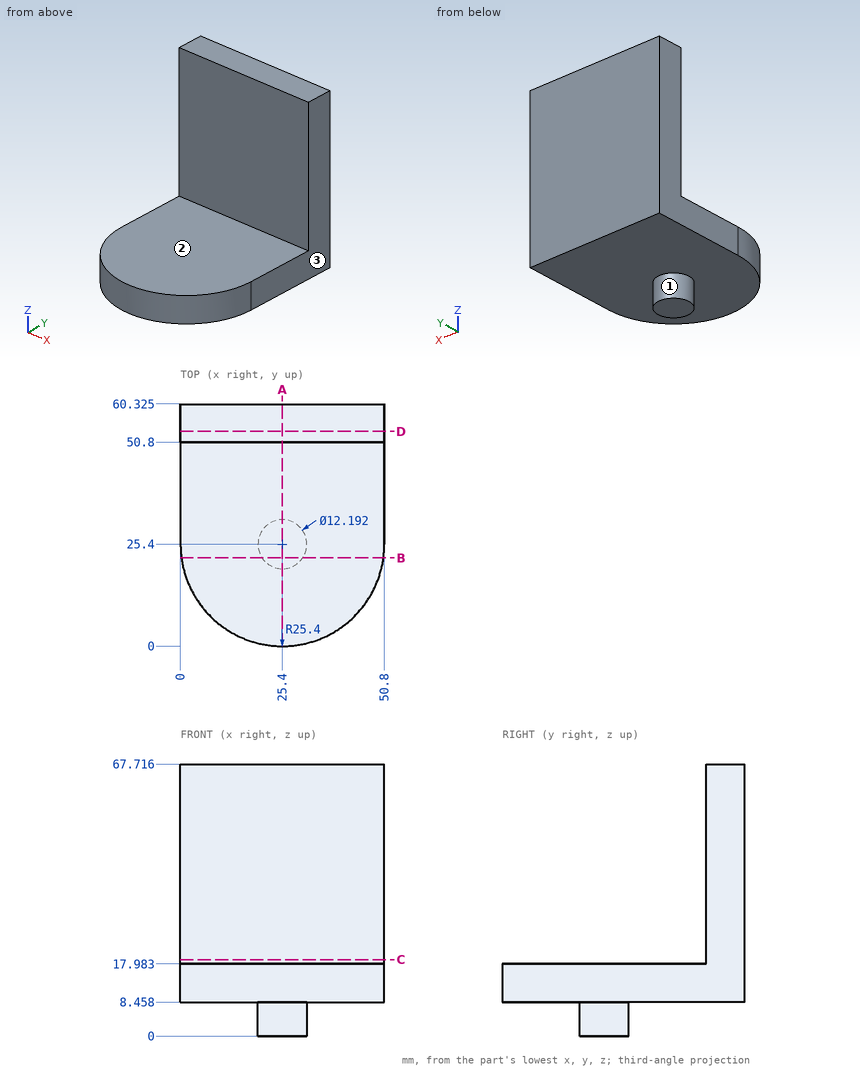
The drawing under review shows one solid part. Ordinate dimensions are in mm from its lowest x, y, z. A direction names the side the tool comes from. Round coordinates to 2 decimals unless told otherwise and drop trailing zeros. Write each loop counter-clockwise with the first axis right and the second up, starting at its lowest first coordinate (ties: lowest second). Pieces come first, ordered by that corner, then holes. Notation, with made-up numbers: M -16.75,26 L 42.25,26 A6 ccw 42.25,30 Z; hole C 29.25,-24 d8. An arc over 180 degrees is marked long. One line per item, written item: value. Start each with the question number.
(1) We need section B-B (y = 22). Give the boundary of the cut face in (x, z).
(2) We need section A-A (x = 25.4). Give the boundary of the cut face in (y, z) (1 decimal), and give its area (3 significant figures).
(3) Wall thickness on line 1 (Y direction, x = 32.5, z = 60) (1 decimal); line 2 (Z direction, x = 39, y = 14.5); line 3 (Z direction, x = 18, y = 56): over which ranges is each line inside the solid? List them lowest first.
(4) Machinability: for the marked faces 1, 2 and 3, which of the approach directions +Z, -Z, +X, -X, +Y, -Y give a long, thin tool a straight path to every point of the face, cutting with its end or side? Answer none if there is none.
(5) We need section D-D (y = 53.5). Give the boundary of the cut face in (x, z).
(6) We need section C-C (z = 19). Give the boundary of the cut face in (x, y) (1 decimal).
(7) Insertion check: pin 1 (1 mm diameter, centred on x = 27, z = 10.5, fed in from -Y); pin 2 (5 mm diameter, centred on x = 19.5, z = 32.5, fed in from -Y); pin 3 (3 mm diameter, centred on x = 28, y = 21, fed in from +Z). Each pin has a flat end and moves straight along its axis. Give the tip position at first contact, or say it passes through.
Result:
1. outline: M 0.23,8.46 L 20.34,8.46 L 20.34,0 L 30.46,0 L 30.46,8.46 L 50.57,8.46 L 50.57,17.98 L 0.23,17.98 Z
2. outline: M 0,8.5 L 19.3,8.5 L 19.3,0 L 31.5,0 L 31.5,8.5 L 60.3,8.5 L 60.3,67.7 L 50.8,67.7 L 50.8,18 L 0,18 Z
2. area: 1,150 mm²
3. line 1: 50.8 to 60.3
3. line 2: 8.46 to 17.98
3. line 3: 8.46 to 67.72
4. face 1: -Z
4. face 2: +Z, +X, -X, -Y
4. face 3: +Z, -Z, +X, +Y, -Y
5. outline: M 0,8.46 L 50.8,8.46 L 50.8,67.72 L 0,67.72 Z
6. outline: M 0,50.8 L 50.8,50.8 L 50.8,60.3 L 0,60.3 Z
7. pin 1: y = 0.02
7. pin 2: y = 50.8
7. pin 3: z = 17.98
